```python
from build123d import *

# Parameters (mm, degrees)
SKETCH1_R               = 4.3
SKETCH1_W               = 12.5
SKETCH1_H               = 12.5
BOSS_EXTRUDE1_DEPTH     = 8
CUT_EXTRUDE1_DEPTH      = 8
SKETCH1_2_R             = 4.3
SKETCH1_2_W             = 12.5
SKETCH1_2_H             = 12.5
BOSS_EXTRUDE2_DEPTH     = 10
CUT_EXTRUDE2_DEPTH      = 3
CUT_EXTRUDE2_DEPTH_BACK = 9
SKETCH3_W               = 12.5
SKETCH3_H               = 12.5
BOSS_EXTRUDE3_DEPTH     = 2
SKETCH4_R               = 4.3
BOSS_EXTRUDE5_DEPTH     = 2
BOSS_EXTRUDE6_DEPTH     = 10
BOSS_EXTRUDE7_DEPTH     = 10
BOSS_EXTRUDE8_DEPTH     = 10
SKETCH8_W               = 18.12209128
SKETCH8_H               = 22.505010211
SKETCH8_W_2             = 16.915072938
SKETCH8_H_2             = 18.768490124
BOSS_EXTRUDE9_DEPTH     = 10
SKETCH12_W              = 16.5
SKETCH12_H              = 16.5
CUT_EXTRUDE6_DEPTH      = 7
SKETCH13_R              = 3.5
CUT_EXTRUDE7_DEPTH      = 7
CUT_EXTRUDE11_DEPTH     = 5


with BuildPart() as part:
    # Sketch1 → Boss-Extrude1 (new body)
    with BuildSketch(Plane.XY):
        with BuildLine():
            Line((-85.345346062, -25.7), (87.254653938, -25.7))
            Line((87.254653938, -25.7), (87.254653938, 0))
            ThreePointArc((87.254653938, 0), (85.409426659, 4.454772721), (80.954653938, 6.3))
            Line((80.954653938, 6.3), (-79.045346062, 6.3))
            ThreePointArc((-79.045346062, 6.3), (-83.500118784, 4.454772721), (-85.345346062, 0))
            Line((-85.345346062, 0), (-85.345346062, -25.7))
        make_face()
        with Locations((-79.045346062, 0)):
            Circle(SKETCH1_R, mode=Mode.SUBTRACT)
        with Locations((80.954653938, 0)):
            Circle(SKETCH1_R, mode=Mode.SUBTRACT)
        with Locations((-77.095346062, -17.45)):
            Rectangle(SKETCH1_W, SKETCH1_H, mode=Mode.SUBTRACT)
        with Locations((79.004653938, -17.45)):
            Rectangle(SKETCH1_W, SKETCH1_H, mode=Mode.SUBTRACT)
    extrude(amount=BOSS_EXTRUDE1_DEPTH)

    # Sketch2 → Cut-Extrude1 (cut)
    with BuildSketch(Plane.XY.offset(8)):
        with BuildLine():
            Line((-35.345346062, 3.5), (37.254653938, 3.5))
            ThreePointArc((37.254653938, 3.5), (40.754653938, 0), (37.254653938, -3.5))
            Line((37.254653938, -3.5), (-35.345346062, -3.5))
            ThreePointArc((-35.345346062, -3.5), (-38.845346062, 0), (-35.345346062, 3.5))
        make_face()
        with BuildLine():
            Line((-35.345346062, -13.95), (37.254653938, -13.95))
            ThreePointArc((37.254653938, -13.95), (40.754653938, -17.45), (37.254653938, -20.95))
            Line((37.254653938, -20.95), (34.643207431, -20.95))
            Line((34.643207431, -20.95), (-35.345346062, -20.95))
            ThreePointArc((-35.345346062, -20.95), (-38.845346062, -17.45), (-35.345346062, -13.95))
        make_face()
    extrude(amount=-CUT_EXTRUDE1_DEPTH, mode=Mode.SUBTRACT)

    # Sketch1<2> → Boss-Extrude2 (add)
    with BuildSketch(Plane.XY):
        with BuildLine():
            Line((-85.345346062, -25.7), (87.254653938, -25.7))
            Line((87.254653938, -25.7), (87.254653938, 0))
            ThreePointArc((87.254653938, 0), (85.409426659, 4.454772721), (80.954653938, 6.3))
            Line((80.954653938, 6.3), (-79.045346062, 6.3))
            ThreePointArc((-79.045346062, 6.3), (-83.500118784, 4.454772721), (-85.345346062, 0))
            Line((-85.345346062, 0), (-85.345346062, -25.7))
        make_face()
        with Locations((-79.045346062, 0)):
            Circle(SKETCH1_2_R, mode=Mode.SUBTRACT)
        with Locations((80.954653938, 0)):
            Circle(SKETCH1_2_R, mode=Mode.SUBTRACT)
        with Locations((-77.095346062, -17.45)):
            Rectangle(SKETCH1_2_W, SKETCH1_2_H, mode=Mode.SUBTRACT)
        with Locations((79.004653938, -17.45)):
            Rectangle(SKETCH1_2_W, SKETCH1_2_H, mode=Mode.SUBTRACT)
    extrude(amount=BOSS_EXTRUDE2_DEPTH)

    # Sketch2<2> → Cut-Extrude2 (cut, two sides)
    with BuildSketch(Plane.XY.offset(8)) as cut_extrude2_sk:
        with BuildLine():
            Line((-35.345346062, 3.5), (37.254653938, 3.5))
            ThreePointArc((37.254653938, 3.5), (40.754653938, 0), (37.254653938, -3.5))
            Line((37.254653938, -3.5), (-35.345346062, -3.5))
            ThreePointArc((-35.345346062, -3.5), (-38.845346062, 0), (-35.345346062, 3.5))
        make_face()
        with BuildLine():
            Line((-35.345346062, -13.95), (37.254653938, -13.95))
            ThreePointArc((37.254653938, -13.95), (40.754653938, -17.45), (37.254653938, -20.95))
            Line((37.254653938, -20.95), (34.643207431, -20.95))
            Line((34.643207431, -20.95), (-35.345346062, -20.95))
            ThreePointArc((-35.345346062, -20.95), (-38.845346062, -17.45), (-35.345346062, -13.95))
        make_face()
    extrude(amount=CUT_EXTRUDE2_DEPTH, mode=Mode.SUBTRACT)
    extrude(cut_extrude2_sk.sketch, amount=-CUT_EXTRUDE2_DEPTH_BACK, mode=Mode.SUBTRACT)

    # Sketch3 → Boss-Extrude3 (add)
    with BuildSketch(Plane.XY.offset(10)):
        with Locations((-77.095346062, -17.45)):
            Rectangle(SKETCH3_W, SKETCH3_H)
        with Locations((79.004653938, -17.45)):
            Rectangle(SKETCH3_W, SKETCH3_H)
    extrude(amount=-BOSS_EXTRUDE3_DEPTH)

    # Sketch4 → Boss-Extrude5 (add)
    with BuildSketch(Plane.XY.offset(10)):
        with Locations((-79.045346062, 0)):
            Circle(SKETCH4_R)
        with Locations((80.954653938, 0)):
            Circle(SKETCH4_R)
    extrude(amount=-BOSS_EXTRUDE5_DEPTH)

    # Sketch5 → Boss-Extrude6 (add)
    with BuildSketch(Plane.XY.offset(10)):
        with BuildLine():
            Line((-4.545346062, 3.5), (6.454653938, 3.5))
            ThreePointArc((6.454653938, 3.5), (2.954653938, 0), (6.454653938, -3.5))
            Line((6.454653938, -3.5), (-4.545346062, -3.5))
            ThreePointArc((-4.545346062, -3.5), (-1.045346062, 0), (-4.545346062, 3.5))
        make_face()
    extrude(amount=-BOSS_EXTRUDE6_DEPTH)

    # Sketch6 → Boss-Extrude7 (add)
    with BuildSketch(Plane.XY.offset(10)):
        with BuildLine():
            Line((-4.545346062, -13.95), (6.454653938, -13.95))
            ThreePointArc((6.454653938, -13.95), (2.954653938, -17.45), (6.454653938, -20.95))
            Line((6.454653938, -20.95), (-4.545346062, -20.95))
            ThreePointArc((-4.545346062, -20.95), (-1.045346062, -17.45), (-4.545346062, -13.95))
        make_face()
    extrude(amount=-BOSS_EXTRUDE7_DEPTH)

    # Sketch7 → Boss-Extrude8 (add)
    with BuildSketch(Plane.XY.offset(10)):
        with BuildLine():
            Line((-85.345346062, -25.7), (-85.345346062, -36.7))
            Line((-85.345346062, -36.7), (-65.345346062, -36.7))
            ThreePointArc((-65.345346062, -36.7), (-62.123520655, -28.921825407), (-54.345346062, -25.7))
            Line((-54.345346062, -25.7), (-85.345346062, -25.7))
        make_face()
        with BuildLine():
            Line((87.254653938, -25.7), (87.254653938, -36.7))
            Line((87.254653938, -36.7), (67.254653938, -36.7))
            ThreePointArc((67.254653938, -36.7), (64.032828531, -28.921825407), (56.254653938, -25.7))
            Line((56.254653938, -25.7), (87.254653938, -25.7))
        make_face()
    extrude(amount=-BOSS_EXTRUDE8_DEPTH)

    # Sketch8 → Boss-Extrude9 (add)
    with BuildSketch(Plane(origin=(0, 0, 0), x_dir=(-1, 0, 0), z_dir=(0, 0, -1))):
        with Locations((-77.426938653, -19.427407937)):
            Rectangle(SKETCH8_W, SKETCH8_H)
        with Locations((75.829945686, -18.535840795)):
            Rectangle(SKETCH8_W_2, SKETCH8_H_2)
    extrude(amount=-BOSS_EXTRUDE9_DEPTH)

    # Sketch12 → Cut-Extrude6 (cut)
    with BuildSketch(Plane(origin=(0, 0, 0), x_dir=(-1, 0, 0), z_dir=(0, 0, -1))):
        with Locations((-77.004653938, -26.45)):
            Rectangle(SKETCH12_W, SKETCH12_H)
        with Locations((75.095346062, -26.45)):
            Rectangle(SKETCH12_W, SKETCH12_H)
    extrude(amount=-CUT_EXTRUDE6_DEPTH, mode=Mode.SUBTRACT)

    # Sketch13 → Cut-Extrude7 (cut)
    with BuildSketch(Plane(origin=(0, 0, 7), x_dir=(-1, 0, 0), z_dir=(0, 0, -1))):
        with Locations((75.095346062, -26.45)):
            Circle(SKETCH13_R)
        with Locations((-77.004653938, -26.45)):
            Circle(SKETCH13_R)
    extrude(amount=-CUT_EXTRUDE7_DEPTH, mode=Mode.SUBTRACT)

    # Sketch14 → Cut-Extrude11 (cut)
    with BuildSketch(Plane(origin=(0, 0, 0), x_dir=(-1, 0, 0), z_dir=(0, 0, -1))):
        with BuildLine():
            Line((-75.954653938, -5.5), (-5.954653938, -5.5))
            ThreePointArc((-5.954653938, -5.5), (-2.729653938, -8.725), (-5.954653938, -11.95))
            Line((-5.954653938, -11.95), (-75.954653938, -11.95))
            ThreePointArc((-75.954653938, -11.95), (-79.179653938, -8.725), (-75.954653938, -5.5))
        make_face()
        with BuildLine():
            Line((4.045346062, -5.5), (6.774875553, -5.5))
            Line((6.774875553, -5.5), (74.045346062, -5.5))
            ThreePointArc((74.045346062, -5.5), (77.270346062, -8.725), (74.045346062, -11.95))
            Line((74.045346062, -11.95), (4.045346062, -11.95))
            ThreePointArc((4.045346062, -11.95), (0.820346062, -8.725), (4.045346062, -5.5))
        make_face()
    extrude(amount=-CUT_EXTRUDE11_DEPTH, mode=Mode.SUBTRACT)


solid = part.part
```
Model file for the job. Use its own axes, mm. A direction names the side the tool comes from. Round coordinates to 2 decimals unless told otherwise and drop trailing zeros. Order: outer loops, then holes, each group sorted by start corner. A loop starts at its lowest first (then second) coordinate and runs counter-clockwise, first axis right, second up. Notation, with made-up numbers: (22.5, -18) -> (68.5, -18) arc R17 cw to (68.5, 8) -> close; hole circle Ø8 at (57.25, 26). An arc over 180 degrees is marked (long way). Use one line per item in the form item = value.
Item 1: Pull direction X, two halves, no side cores. Call faces 1 (the face through (85.255, -27, 3)), 2 (the face through (2, 6.3, 5)): released by +X, released by -X, zero draft, split by the parting line, or undercut.
Returned:
face_1 = undercut
face_2 = zero draft
Item 2: Cut at A-A, the plane x = 17.5. Write the cut outline in (y, z).
Returned:
outline = (-25.7, 0) -> (-20.95, 0) -> (-20.95, 10) -> (-25.7, 10) -> close; (-13.95, 0) -> (-11.95, 0) -> (-11.95, 5) -> (-5.5, 5) -> (-5.5, 0) -> (-3.5, 0) -> (-3.5, 10) -> (-13.95, 10) -> close; (3.5, 0) -> (6.3, 0) -> (6.3, 10) -> (3.5, 10) -> close
Item 3: Drill centre lines: line 1 (Y direction, x = -20, z = 6.5); line 2 (X direction, y = -0.5, z = 1); line 3 (Y direction, x = 34.5, z = 3.5). Where is each one in solid material? Low to high.
Returned:
line_1 = -25.7 to -20.95, -13.95 to -3.5, 3.5 to 6.3
line_2 = -85.35 to -83.32, -74.77 to -38.81, -1.08 to 2.99, 40.72 to 76.68, 85.23 to 87.25
line_3 = -25.7 to -20.95, -13.95 to -11.95, -5.5 to -3.5, 3.5 to 6.3
Item 4: Cut at B-B, the plane y = -2. Write the cut outline in (x, z), and give its area (3 significant figures).
Returned:
outline = (-85.35, 0) -> (-82.85, 0) -> (-82.85, 8) -> (-75.24, 8) -> (-75.24, 0) -> (-38.22, 0) -> (-38.22, 10) -> (-85.35, 10) -> close; (-1.67, 0) -> (3.58, 0) -> (3.58, 10) -> (-1.67, 10) -> close; (40.13, 0) -> (77.15, 0) -> (77.15, 8) -> (84.76, 8) -> (84.76, 0) -> (87.25, 0) -> (87.25, 10) -> (40.13, 10) -> close
area = 873 mm^2
Item 5: Flat gauge pins, fed straight in: pin 1 Ø1.5 at (x, z) = (-46.5, 2) entering from -Y; pin 2 Ø5 at (x, y) = (-43, -10) entering from -Z; pin 3 Ø8 at (x, y) = (-75.5, -22.5) entering from -Z; pin 4 Ø5 at (x, y) = (-9, -29.5) entering from -Z. Where does each tip first touch, or does it go through?
Returned:
pin_1 = -25.7
pin_2 = 0
pin_3 = 7
pin_4 = through
Item 6: Tool access for faces 3 (the face through (64.12, -29.01, 5.07)), 4 (the face through (-75, -36.7, 5)), 5 (the face through (-20, 3.5, 5)), 6 (the face through (-40, -11.95, 2)): list every direction of +Z, -Z, +X, -X, +Y, -Y with a clear straight run to the whole face (end or side of a thin tool).
Returned:
face_3 = +Z, -Z, -Y
face_4 = +Z, -Z, +X, -X, -Y
face_5 = +Z, -Z
face_6 = -Z
